Geometry check sheet. Reference: the model listing, model coordinates, mm. A direction names the side the tool comes from. Give positions to 0.01 mm unless a question says otherwise; leave off trailing zeros. Write each loop counter-clockwise with the first axis right and the second up, starting at its lowest first coordinate (ties: lowest second). Pieces come first, ordered by that corner, then holes. Notation, with made-up numbers: (38.25, 32) - (79.25, 32) arc R10 ccw to (79.25, 41) - close; hole circle Ø11 at (73.5, 21). An arc over 180 degrees is marked (long way). Write item = value, one per line. Start each with the question number.
(1) Depth check by flat-ended pin: pin 1 Ø2 at (x, z) = (-91, -107.5) entering from -Y; pin 2 Ø8 at (y, z) = (-81.5, -4) entering from +X; pin 3 Ø3 at (y, z) = (43.5, -89.5) entering from -X. Enter the tip coordinate at first touch or a pass-through.
(2) Draft check along Z on faces 1 (the conical face through (-30.228, -136.127, -4.111)), 2 (the conical face through (108.97, 106.28, 124.99)), 3 (the flat face through (-90, 108, 1)). Enter one of: pulls with the +Z half, pulls with the -Z half, needs draft (parallel to the pull), parting line crosses it, or undercut.
(3) Thickness scan on L1, parallel to Z at x = -42, y = 1; L2, parallel to Z at x = -126, y = 91; L3, parallel to X at y = 98, z = -52. Record the ranges inside material, lowest first.
(4) Section check A-A, the plane y = 0. Enter the section's corners in (x, z), plus the area to 3 significant figures.
(5) Section check D-D, the plane z = 86. Enter the section's corners in (x, y).
(6) Section check B-B, the plane x = 0. Enter the section's corners in (y, z), plus the area to 3 significant figures.
(7) Access from +Z, -Z, +X, -X, +Y, -Y to the whole of each face (thin tool, end or side, straight path). Record for faces 4 (the conical face through (102.784, 100.339, -125.013)), 5 (the cylindrical face through (107.5, 104.2, -140.5)).
```python
from build123d import *

# Parameters (mm, degrees)
TAPERED_PAIL_BLANK_START  = -190
PAIL_BASE_PROFILE_R       = 135
TAPERED_PAIL_BLANK_DEPTH  = 375
TAPERED_PAIL_BLANK_DRAFT  = -1.985458585
PAIL_WALL_2MM_T           = -2
PAIL_REINFORCED_RIM_START = 177
PAIL_RIM_PROFILE_R        = 158
PAIL_RIM_PROFILE_R_2      = 146
PAIL_REINFORCED_RIM_DEPTH = 8
LOADING_OPENING_PROFILE_W = 220
LOADING_OPENING_PROFILE_H = 250
TOP_LOADING_OPENING_DEPTH = 90


with BuildPart() as part:
    # Pail_Base_Profile → Tapered_Pail_Blank (with draft: the straight prism first)
    with BuildSketch(Plane.XY.offset(TAPERED_PAIL_BLANK_START)):
        Circle(PAIL_BASE_PROFILE_R)
    extrude(amount=TAPERED_PAIL_BLANK_DEPTH)
    # Tapered_Pail_Blank: the draft: its side faces are tilted about the plane it starts from
    tapered_pail_blank_sides = [part.faces().sort_by_distance(p)[0] for p in [
        (-135, 0, -2.5),
    ]]
    draft(tapered_pail_blank_sides, Plane.XY.offset(TAPERED_PAIL_BLANK_START), TAPERED_PAIL_BLANK_DRAFT)

    # Pail_Wall_2mm
    pail_wall_2mm_openings = [part.faces().sort_by_distance(p)[0] for p in [
        (0, 0, 185),
    ]]
    offset(amount=PAIL_WALL_2MM_T, openings=pail_wall_2mm_openings, kind=Kind.INTERSECTION)

    # Pail_Rim_Profile → Pail_Reinforced_Rim (add)
    with BuildSketch(Plane.XY.offset(PAIL_REINFORCED_RIM_START)):
        Circle(PAIL_RIM_PROFILE_R)
        Circle(PAIL_RIM_PROFILE_R_2, mode=Mode.SUBTRACT)
    extrude(amount=PAIL_REINFORCED_RIM_DEPTH)

    # Loading_Opening_Profile → Top_Loading_Opening (cut, symmetric)
    with BuildSketch(Plane(origin=(0, 0, 0), x_dir=(0, 0, -1), z_dir=(1, 0, 0))):
        with Locations((0, 125)):
            Rectangle(LOADING_OPENING_PROFILE_W, LOADING_OPENING_PROFILE_H)
    extrude(amount=TOP_LOADING_OPENING_DEPTH, both=True, mode=Mode.SUBTRACT)

    # Drum_Hinge_Knuckle_Profile → Drum_Hinge_Knuckles (revolve)
    with BuildSketch(Plane(origin=(0, 0, 0), x_dir=(0, 0, 1), z_dir=(0.6974653404967203, -0.7166185169291917, 0)), mode=Mode.PRIVATE) as drum_hinge_knuckles_sk:
        Polygon((-155, -142.213651728), (-125.000089364, -143.255770649), (-125.243089364, -150.251112671), (-155.243, -149.208993749), align=None)
        Polygon((125, -151.920290486), (154.999910636, -152.962409408), (154.756910636, -159.95775143), (124.757, -158.915632508), align=None)
    revolve(drum_hinge_knuckles_sk.sketch.rotate(Axis((101.521807726, 98.808418315, -169.999121159), (0.024888838213313905, 0.024223630298311177, 0.9993966987475805)), 210.380878097), axis=Axis((101.521807726, 98.808418315, -169.999121159), (0.024888838213313905, 0.024223630298311177, 0.9993966987475805)))


solid = part.part
```
Model answer:
q1.pin_1 = -104.43
q1.pin_2 = 118.33
q1.pin_3 = -131.96
q2.face_1 = pulls with the +Z half
q2.face_2 = undercut
q2.face_3 = needs draft
q3.L1 = -190 to -188
q3.L2 = 177 to 185
q3.L3 = -99.68 to -96.85, 96.85 to 99.68
q4.outline = (-158, 177) - (-147.72, 177) - (-135, -190) - (135, -190) - (147.72, 177) - (158, 177) - (158, 185) - (146, 185) - (133.07, -188) - (-133.07, -188) - (-146, 185) - (-158, 185) - close
q4.area = 2,200 mm²
q5.outline = (-90, 110.57) - (-90, 113.14) arc R144.57 ccw (long way) to (90, 113.14) - (90, 110.57) arc R142.57 cw (long way) to start
q6.outline = (-158, 177) - (-147.72, 177) - (-135, -190) - (135, -190) - (137.77, -110) - (135.77, -110) - (133.07, -188) - (-133.07, -188) - (-146, 185) - (-158, 185) - close; (143.4, 110) - (145.4, 110) - (147.72, 177) - (158, 177) - (158, 185) - (146, 185) - close
q6.area = 1,750 mm²
q7.face_4 = +X, +Y
q7.face_5 = none
